```python
from build123d import *

# Parameters (mm, degrees)
F0_R     = 5
F0_R_2   = 3
F1_DEPTH = 2.5
F2_R     = 5
F2_R_2   = 3
F3_DEPTH = 2.5
F5_DEPTH = 2.5


with BuildPart() as f1:
    # F0 (on Front) → F1 (new body)
    with BuildSketch(Plane.XZ):
        Circle(F0_R)
        Circle(F0_R_2, mode=Mode.SUBTRACT)
    extrude(amount=F1_DEPTH)



with BuildPart() as f3:
    # F2 (on Front) → F3 (new body)
    with BuildSketch(Plane.XZ):
        with Locations((11.5, 0)):
            Circle(F2_R)
        with Locations((11.5, 0)):
            Circle(F2_R_2, mode=Mode.SUBTRACT)
    extrude(amount=F3_DEPTH)


with BuildPart() as f1_1:
    add(f1.part)

    add(f3.part)  # F5 merges F3
    # F4 (on face) → F5 (join)
    with BuildSketch(Plane.XZ.offset(2.5)):
        with BuildLine():
            ThreePointArc((8.4708627887, 3.8414155761), (5.8357068684, 3.1228084753), (3.2005509482, 3.8414155761))
            ThreePointArc((3.2005509482, 3.8414155761), (5, 0), (3.2005509482, -3.8414155761))
            ThreePointArc((3.2005509482, -3.8414155761), (5.8357068684, -3.1228084753), (8.4708627887, -3.8414155761))
            ThreePointArc((8.4708627887, -3.8414155761), (6.6079507491, 0), (8.4708627887, 3.8414155761))
        make_face()
    extrude(amount=-F5_DEPTH)


solid = f1_1.part
```
For this review, take the finished solid that the model builds, in its own axes (mm). Round coordinates to 2 decimals unless told otherwise and drop trailing zeros. Write each loop counter-clockwise with the first axis right and the second up, starting at its lowest first coordinate (ties: lowest second). Pieces come first, ordered by that corner, then holes. Notation, with made-up numbers: (33, -33.5) - (85, -33.5) arc R21 cw to (85, -9.5) - close; hole circle Ø2 at (60, -7.75). An arc over 180 degrees is marked (long way). Write each question's results on one line, items separated by ' | '.
Item 1: Take a section at C-C on x = 11. State the section outline as (y, z) points.
Calculated:
outline: (-2.5, -4.97) - (0, -4.97) - (0, -2.96) - (-2.5, -2.96) - close; (-2.5, 2.96) - (0, 2.96) - (0, 4.97) - (-2.5, 4.97) - close
Item 2: Take a section at D-D on z = -2.5. State the section outline as (x, y) points.
Calculated:
outline: (-4.33, -2.5) - (-1.66, -2.5) - (-1.66, 0) - (-4.33, 0) - close; (1.66, -2.5) - (9.84, -2.5) - (9.84, 0) - (1.66, 0) - close; (13.16, -2.5) - (15.83, -2.5) - (15.83, 0) - (13.16, 0) - close
Item 3: Draft analysis for pull direction X (two halves, no side actions). For faces 1 (the face through (6, -2.5, 0)), 2 (the face through (5.56, -1.27, -3.13)), state which applies: pulls with the +X half, pulls with the -X half, needs draft (parallel to the pull), parting line crosses it, or undercut.
Calculated:
face 1: needs draft | face 2: undercut
Item 4: To check wall thickness, follow line 1 along Z through (x, y) = (11.5, -0.65); line 2 along X through (y, z) = (-0.2, -2.75); line 3 along X through (y, z) = (-0.8, 2.25). State the ranges of each line that lie inside material, in increasing order. Write a range as from..to.
Calculated:
line 1: z = -5..-3, 3..5 | line 2: x = -4.18..-1.2, 1.2..10.3, 12.7..15.68 | line 3: x = -4.47..-1.98, 1.98..9.52, 13.48..15.97
Item 5: Take a section at A-A on z = 0. State the section outline as (x, y) points.
Calculated:
outline: (-5, -2.5) - (-3, -2.5) - (-3, 0) - (-5, 0) - close; (3, -2.5) - (8.5, -2.5) - (8.5, 0) - (3, 0) - close; (14.5, -2.5) - (16.5, -2.5) - (16.5, 0) - (14.5, 0) - close
Item 6: For pin 1 (1.5 mm diameter, centred on y = -1.5, z = 1, fed in from -X); pin 2 (1.5 mm diameter, centred on y = -1, z = 3.5, fed in from -X); pin 3 (1 mm diameter, centred on x = -2, y = -2, fed in from +Z), all flat-tipped, find the tip position at first contact; note any pin that passes through.
Calculated:
pin 1: stops at x = -4.99 | pin 2: stops at x = -4.18 | pin 3: stops at z = 4.77
Item 7: Take a section at B-B on x = 0. State the section outline as (y, z) points, then the cut area to 3 significant figures.
Calculated:
outline: (-2.5, -5) - (0, -5) - (0, -3) - (-2.5, -3) - close; (-2.5, 3) - (0, 3) - (0, 5) - (-2.5, 5) - close | area: 10.0 mm^2
